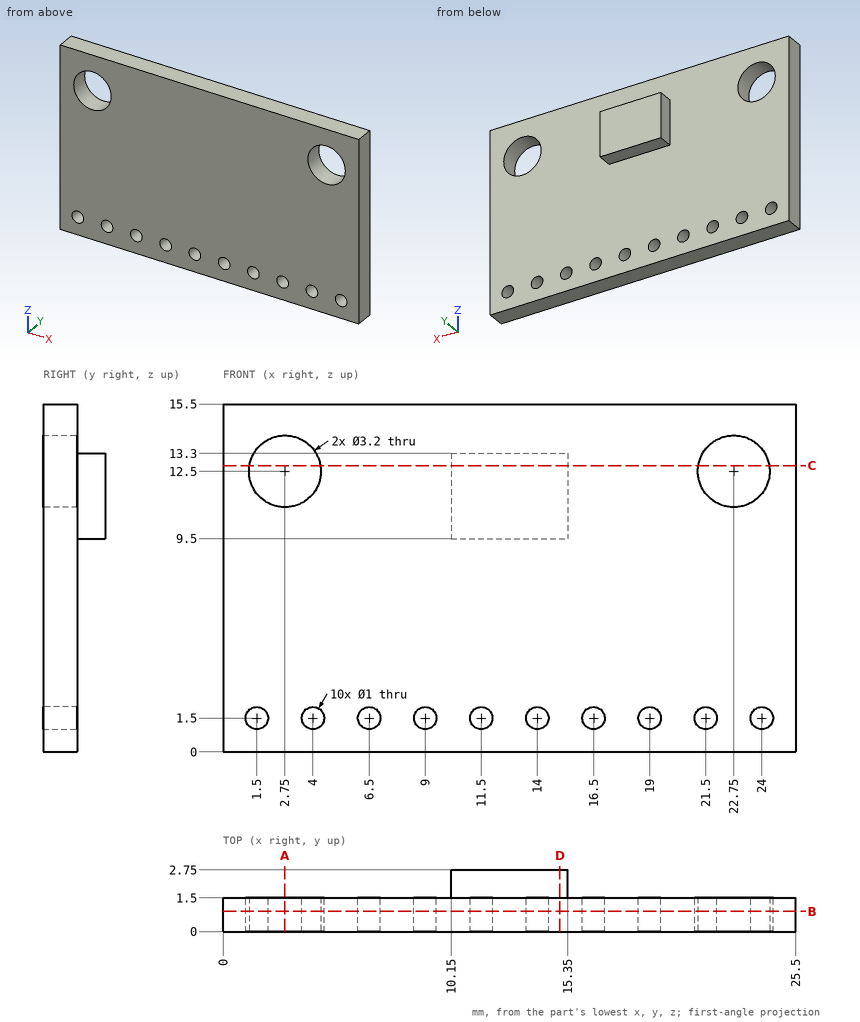
The figure shows three views and two pictorial views of one solid part (mm, origin at its lowest corner). Answer the questions. Coordinates: 2 decimals unless noted, no trailing zeros. Loops run counter-clockwise (first coordinate to the right, second up) from the corner with the lowest first, then second, coordinate; pieces in that order, holes last. Notation, with made-up numbers: (13, 38.25) -> (51, 38.25) arc R17 cw to (51, 52.25) -> close; hole circle Ø8 at (-5, 23). An arc over 180 degrees is marked (long way). Return JSON: item names as keys, results as strings. Group by question number.
(1) A cutting plane is placed at D-D on x = 15. Write down the section's boundary in (y, z).
(2) A cutting plane is placed at C-C on z = 12.75. Write down the section's boundary in (x, y).
(3) A cutting plane is placed at A-A on x = 2.75. Write down the section's boundary in (y, z).
(4) A cutting plane is placed at B-B on y = 0.9. Count the separate pieces of the cut face and the enclosed holes in it, and give its area (3 significant figures).
(5) Find the intervals of material crossed by probe 1 along Z at (x, y) = (21.75, 1.2); probe 2 along Z at (x, y) = (24, 0.55); probe 3 along Y at (x, z) = (12, 7.25), in increasing order. Write a range as from..to.
(6) Given pin 1 Ø3.5 at (x, z) = (2.75, 12.5) entering from +Y; pin 2 Ø0.6 at (x, y) = (13.5, 2) entering from +Z, each flat-ended and moving along its own axis, determine where each tip first touches the part or whether it passes through.
The answers:
{
 "1": {"outline": "(0, 0) -> (1.5, 0) -> (1.5, 9.5) -> (2.75, 9.5) -> (2.75, 13.3) -> (1.5, 13.3) -> (1.5, 15.5) -> (0, 15.5) -> close"},
 "2": {"outline": "(0, 0) -> (1.17, 0) -> (1.17, 1.5) -> (0, 1.5) -> close; (4.33, 0) -> (21.17, 0) -> (21.17, 1.5) -> (15.35, 1.5) -> (15.35, 2.75) -> (10.15, 2.75) -> (10.15, 1.5) -> (4.33, 1.5) -> close; (24.33, 0) -> (25.5, 0) -> (25.5, 1.5) -> (24.33, 1.5) -> close"},
 "3": {"outline": "(0, 0) -> (1.5, 0) -> (1.5, 10.9) -> (0, 10.9) -> close; (0, 14.1) -> (1.5, 14.1) -> (1.5, 15.5) -> (0, 15.5) -> close"},
 "4": {"separate pieces": "1", "enclosed holes": "12", "area": "371 mm^2"},
 "5": {"probe 1": "z = 0..1.07, 1.93..11.25, 13.75..15.5", "probe 2": "z = 0..1, 2..11.5, 13.5..15.5", "probe 3": "y = 0..1.5"},
 "6": {"pin 1": "stops at y = 1.5", "pin 2": "stops at z = 13.3"}
}
